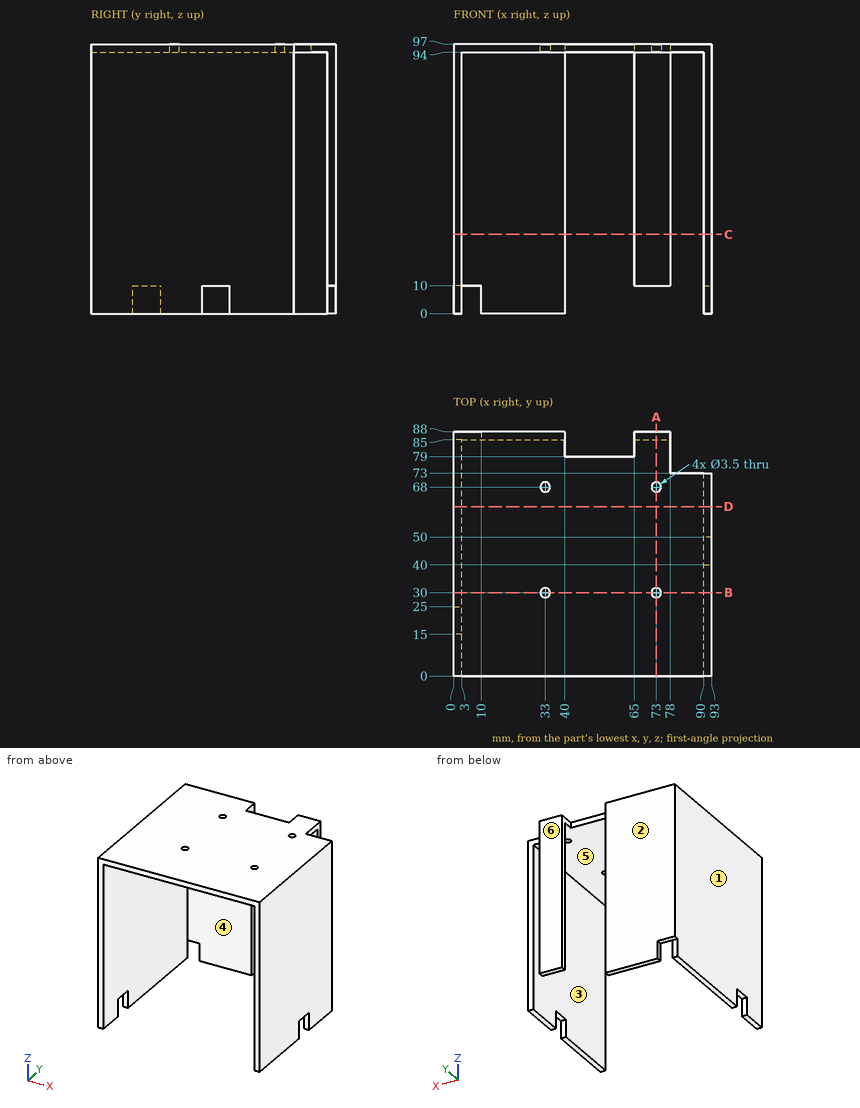
Geometry check sheet. Reference: drawing and pictorial views, mm from the part's lowest x, y, z. A direction names the side the tool comes from. Coordinates: 2 decimals unless noted, no trailing zeros. Order: outer loops, then holes, each group sorted by start corner. A loop starts at its lowest first (then second) coordinate and runs counter-clockwise, first axis right, second up. Notation, with made-up numbers: (-33, 12) -> (-29, 12) arc R30 cw to (-29, 39) -> close; hole circle Ø1 at (39, 62.25). An arc over 180 degrees is marked (long way). Put each result on its own line as item: value. Start each with the question number.
1) Release check for a two-part mould opening along X. For the marked faces 1, 2 and 3 record: pulls with the +X half, pulls with the -X half, needs draft (parallel to the pull), parting line crosses it, or undercut.
2) Cross-section at A-A (x = 73). Enter the section's corners in (y, z).
3) Cross-section at B-B (y = 30). Enter the section's corners in (x, z), plus the area to 3 significant figures.
4) Cross-section at C-C (z = 28.5). Enter the section's corners in (x, y).
5) Tool access check on the marked faces 4, 5 and 6. Record the directions out of +Z, -Z, +X, -X, +Y, -Y that give a thin tool (end or side, any length) a straight path to the whole face; none if there is none.
6) Go/stop test with flat-tipped pins: pin 1 (4.5 mm diameter, centred on x = 89, z = 68, fed in from +Y); pin 2 (1.5 mm diameter, centred on x = 17, z = 37, fed in from -Y); pin 3 (16.5 mm diameter, centred on y = 83, z = 73, fed in from +X); pin 4 (3 mm diameter, centred on x = 33, y = 68, fed in from +Z). Record where each tip stops, or that it passes through.
7) Cross-section at D-D (y = 61). Enter the section's corners in (x, z).
8) Material ranges on L1, parallel to X at y = 68, z = 96; L2, parallel to Y at x = 73, z = 95; L3, parallel to X at y = 37, z = 7.5, recorded low to high.
Geometry check:
1. face 1: pulls with the -X half
1. face 2: needs draft
1. face 3: undercut
2. outline: (0, 94) -> (28.25, 94) -> (28.25, 97) -> (0, 97) -> close; (31.75, 94) -> (66.25, 94) -> (66.25, 97) -> (31.75, 97) -> close; (69.75, 94) -> (85, 94) -> (85, 10) -> (88, 10) -> (88, 97) -> (69.75, 97) -> close
3. outline: (0, 0) -> (3, 0) -> (3, 94) -> (31.25, 94) -> (31.25, 97) -> (0, 97) -> close; (34.75, 94) -> (71.25, 94) -> (71.25, 97) -> (34.75, 97) -> close; (74.75, 94) -> (90, 94) -> (90, 0) -> (93, 0) -> (93, 97) -> (74.75, 97) -> close
3. area: 822 mm^2
4. outline: (0, 0) -> (3, 0) -> (3, 85) -> (40, 85) -> (40, 88) -> (0, 88) -> close; (65, 85) -> (78, 85) -> (78, 88) -> (65, 88) -> close; (90, 0) -> (93, 0) -> (93, 73) -> (90, 73) -> close
5. face 4: -Z, +X, -Y
5. face 5: -Z, -Y
5. face 6: +Z, -Z, +X, -X, +Y
6. pin 1: stops at y = 73
6. pin 2: stops at y = 85
6. pin 3: stops at x = 78
6. pin 4: passes through
7. outline: (0, 0) -> (3, 0) -> (3, 94) -> (90, 94) -> (90, 0) -> (93, 0) -> (93, 97) -> (0, 97) -> close
8. L1: x = 0 to 31.25, 34.75 to 71.25, 74.75 to 93
8. L2: y = 0 to 28.25, 31.75 to 66.25, 69.75 to 88
8. L3: x = 0 to 3, 90 to 93
